Can you work these out from the model? Positions are in its coordinate system, mm. Round coordinates to 2 decimals unless told otherwise and drop trailing zeros. Loops run counter-clockwise (first coordinate to the right, second up) from the corner with the lowest first, then second, coordinate; pieces in that order, holes last.
(1) I want a section at D-D on y = 2.25. Give the number of separate pieces and of enclosed holes in the cut face, plus the area to 3 significant figures.
(2) I want a section at B-B on x = -43. Write out the boundary of the cut face in (y, z), plus the area to 3 significant figures.
(3) Will these pins go through, and if not, where does the flat tip stop? pin 1 Ø6.5 at (x, z) = (33, -45.5) entering from -Y; pin 2 Ø1.5 at (x, y) = (21.5, 4.5) entering from +Z; pin 3 Ø1 at (y, z) = (2, -39) entering from -X.
(4) If I drill on line 1 along X through (y, z) = (1.5, 0); line 2 along X through (y, z) = (2.75, -42.5); line 3 along X through (y, z) = (5, 57.5) (3 decimals), over which ranges is the centre line in solid material (lowest first)?
(5) I want a section at A-A on z = -22.5. Write out the boundary of the cut face in (x, y).
(6) I want a section at C-C on z = 48. Write out the boundary of the cut face in (x, y), plus the area to 3 significant figures.
from build123d import *

# Parameters (mm, degrees)
SKETCH1_R                       = 85
SKETCH1_R_2                     = 2.5
SKETCH1_R_3                     = 2
BOSS_EXTRUDE1_DEPTH             = 6.35
CBORE_FOR_M3_SHCS1_D            = 3.3
CBORE_FOR_M3_SHCS1_CBORE_D      = 8
CBORE_FOR_M3_SHCS1_CBORE_DEPTH  = 3.5
CBORE_FOR_M3_SHCS2_D            = 3.3
CBORE_FOR_M3_SHCS2_CBORE_D      = 8
CBORE_FOR_M3_SHCS2_CBORE_DEPTH  = 3.5
CBORE_SLOT_FOR_M3_SHCS1_DEPTH   = 3.5
CBORE_START                     = 3.5
CBORE_SLOT_FOR_M3_SHCS1_2_DEPTH = 2.85
CBORE_SLOT_FOR_M3_SHCS2_DEPTH   = 3.5
CBORE_SLOT_FOR_M3_SHCS2_2_DEPTH = 2.85
SKETCH16_R                      = 1.65
CUT_EXTRUDE1_DEPTH              = 1


# Read off the part's stored shape, not the designer's step: CBORE SLOT for M3 SHCS1, CBORE SLOT for M3 SHCS2
with BuildPart() as part:
    # Sketch1 → Boss-Extrude1 (new body)
    with BuildSketch(Plane(origin=(0, 0, 0), x_dir=(1, 0, 0), z_dir=(0, 1, 0))):
        with Locations(Location((0, 0, 0), (0, 0, 270))):
            Circle(SKETCH1_R)
        with Locations(Location((0, 0, 0), (0, 0, 270))):
            Circle(SKETCH1_R_2, mode=Mode.SUBTRACT)
        with Locations(Location((-31.48, 12.25, 0), (0, 0, 270))):
            Circle(SKETCH1_R_3, mode=Mode.SUBTRACT)
        with BuildLine():
            Line((-38, 62.329768169), (-38, -62.329768169))
            ThreePointArc((-38, -62.329768169), (-49.900096859, -53.282082668), (-59.707620954, -42))
            Line((-59.707620954, -42), (-59.707620954, 42))
            ThreePointArc((-59.707620954, 42), (-49.900096859, 53.282082668), (-38, 62.329768169))
        make_face(mode=Mode.SUBTRACT)
        with BuildLine():
            Line((38, 62.329768169), (38, -62.329768169))
            ThreePointArc((38, -62.329768169), (49.900096859, -53.282082668), (59.707620954, -42))
            Line((59.707620954, -42), (59.707620954, 42))
            ThreePointArc((59.707620954, 42), (49.900096859, 53.282082668), (38, 62.329768169))
        make_face(mode=Mode.SUBTRACT)
    extrude(amount=BOSS_EXTRUDE1_DEPTH)

    # CBORE for M3 SHCS1 (through all)
    with Locations(Plane(origin=(0, 0, 0), x_dir=(-1, 0, 0), z_dir=(0, -1, 0))):
        with Locations((-33, 5), (-33, -5), (33, 5), (33, -5), (63.157620954, 0), (-63.157620954, 0)):
            CounterBoreHole(CBORE_FOR_M3_SHCS1_D / 2, CBORE_FOR_M3_SHCS1_CBORE_D / 2, CBORE_FOR_M3_SHCS1_CBORE_DEPTH)

    # CBORE for M3 SHCS2 (through all)
    with Locations(Plane(origin=(0, 0, 0), x_dir=(-1, 0, 0), z_dir=(0, -1, 0))):
        with Locations((22.5, -26.887097638), (-22.5, -26.887097638), (22.5, -41.887097638), (-22.5, -41.887097638)):
            CounterBoreHole(CBORE_FOR_M3_SHCS2_D / 2, CBORE_FOR_M3_SHCS2_CBORE_D / 2, CBORE_FOR_M3_SHCS2_CBORE_DEPTH)

    # CBORE SLOT for M3 SHCS1 outline → CBORE SLOT for M3 SHCS1 (cut)
    with BuildSketch(Plane(origin=(0, 0, 0), x_dir=(1, 0, 0), z_dir=(0, 1, 0))):
        with BuildLine():
            ThreePointArc((-30, 58.35), (-34, 62.35), (-38, 58.35))
            Line((-38, 58.35), (-38, 31.65))
            ThreePointArc((-38, 31.65), (-34, 27.65), (-30, 31.65))
            Line((-30, 31.65), (-30, 58.35))
        make_face()
        with BuildLine():
            ThreePointArc((12, 58.35), (8, 62.35), (4, 58.35))
            Line((4, 58.35), (4, 31.65))
            ThreePointArc((4, 31.65), (8, 27.65), (12, 31.65))
            Line((12, 31.65), (12, 58.35))
        make_face()
        with BuildLine():
            ThreePointArc((37, 58.35), (33, 62.35), (29, 58.35))
            Line((29, 58.35), (29, 31.65))
            ThreePointArc((29, 31.65), (33, 27.65), (37, 31.65))
            Line((37, 31.65), (37, 58.35))
        make_face()
    extrude(amount=CBORE_SLOT_FOR_M3_SHCS1_DEPTH, mode=Mode.SUBTRACT)

    # CBORE SLOT for M3 SHCS1 2 outline → CBORE SLOT for M3 SHCS1 2 (cut)
    with BuildSketch(Plane(origin=(0, 0, 0), x_dir=(1, 0, 0), z_dir=(0, 1, 0)).offset(CBORE_START)):
        with BuildLine():
            ThreePointArc((-32.35, 58.35), (-34, 60), (-35.65, 58.35))
            Line((-35.65, 58.35), (-35.65, 31.65))
            ThreePointArc((-35.65, 31.65), (-34, 30), (-32.35, 31.65))
            Line((-32.35, 31.65), (-32.35, 58.35))
        make_face()
        with BuildLine():
            ThreePointArc((9.65, 58.35), (8, 60), (6.35, 58.35))
            Line((6.35, 58.35), (6.35, 31.65))
            ThreePointArc((6.35, 31.65), (8, 30), (9.65, 31.65))
            Line((9.65, 31.65), (9.65, 58.35))
        make_face()
        with BuildLine():
            ThreePointArc((34.65, 58.35), (33, 60), (31.35, 58.35))
            Line((31.35, 58.35), (31.35, 31.65))
            ThreePointArc((31.35, 31.65), (33, 30), (34.65, 31.65))
            Line((34.65, 31.65), (34.65, 58.35))
        make_face()
    extrude(amount=CBORE_SLOT_FOR_M3_SHCS1_2_DEPTH, mode=Mode.SUBTRACT)

    # CBORE SLOT for M3 SHCS2 outline → CBORE SLOT for M3 SHCS2 (cut)
    with BuildSketch(Plane(origin=(0, 0, 0), x_dir=(1, 0, 0), z_dir=(0, 1, 0))):
        with BuildLine():
            ThreePointArc((-28.35, 54), (-29.194001893, 53.909943836), (-30, 53.643830402))
            Line((-30, 53.643830402), (-30, 46.356169598))
            ThreePointArc((-30, 46.356169598), (-29.194001893, 46.090056164), (-28.35, 46))
            Line((-28.35, 46), (-0.65, 46))
            ThreePointArc((-0.65, 46), (3.35, 50), (-0.65, 54))
            Line((-0.65, 54), (-28.35, 54))
        make_face()
    extrude(amount=CBORE_SLOT_FOR_M3_SHCS2_DEPTH, mode=Mode.SUBTRACT)

    # CBORE SLOT for M3 SHCS2 2 outline → CBORE SLOT for M3 SHCS2 2 (cut)
    with BuildSketch(Plane(origin=(0, 0, 0), x_dir=(1, 0, 0), z_dir=(0, 1, 0)).offset(CBORE_START)):
        with BuildLine():
            ThreePointArc((-28.35, 51.65), (-30, 50), (-28.35, 48.35))
            Line((-28.35, 48.35), (-0.65, 48.35))
            ThreePointArc((-0.65, 48.35), (1, 50), (-0.65, 51.65))
            Line((-0.65, 51.65), (-28.35, 51.65))
        make_face()
    extrude(amount=CBORE_SLOT_FOR_M3_SHCS2_2_DEPTH, mode=Mode.SUBTRACT)

    # Sketch16 → Cut-Extrude1 (cut)
    with BuildSketch(Plane.XZ):
        with Locations(Location((0, -70, 0), (0, 0, 270))):
            Circle(SKETCH16_R)
        with Locations(Location((0, 70, 0), (0, 0, 90))):
            Circle(SKETCH16_R)
    extrude(amount=-CUT_EXTRUDE1_DEPTH, mode=Mode.SUBTRACT)


solid = part.part
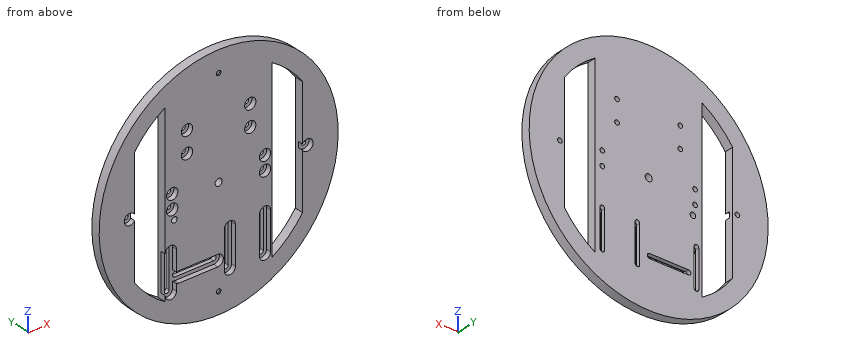
Filled sheet:
1. separate pieces: 1
1. enclosed holes: 14
1. area: 16,500 mm2
2. outline: (0, -73.32) - (6.35, -73.32) - (6.35, -58.99) - (0, -58.99) - close; (0, 58.99) - (6.35, 58.99) - (6.35, 73.32) - (0, 73.32) - close
2. area: 182 mm2
3. pin 1: stops at y = 3.5
3. pin 2: stops at z = 82.43
3. pin 3: stops at x = -75.78
4. line 1: x = -85 to -67.16, -38 to -2.5, 2.5 to 38, 67.16 to 85
4. line 2: x = -73.61 to -59.35, -30 to 4, 12 to 29, 37 to 38, 59.35 to 73.61
4. line 3: x = -62.6 to -44.975, -38 to 38, 44.975 to 62.6
5. outline: (-81.97, 0) - (-59.71, 0) - (-59.71, 6.35) - (-81.97, 6.35) - close; (-38, 0) - (38, 0) - (38, 6.35) - (-38, 6.35) - close; (59.71, 0) - (81.97, 0) - (81.97, 6.35) - (59.71, 6.35) - close
6. outline: (-70.15, 0) - (-55, 0) - (-55, 6.35) - (-70.15, 6.35) - close; (-38, 0) - (38, 0) - (38, 6.35) - (-38, 6.35) - close; (55, 0) - (70.15, 0) - (70.15, 6.35) - (55, 6.35) - close
6. area: 675 mm2
